Autodesk Inventor part; units mm, degrees
ref_plane "YZ Plane" through (0, 0, 0) normal (1, 0, 0) x (0, 1, 0)
ref_plane "XZ Plane" through (0, 0, 0) normal (0, 1, 0) x (-1, 0, 0)
ref_plane "XY Plane" through (0, 0, 0) normal (0, 0, 1) x (1, 0, 0)
sketch "Sketch1" plane through (0, 0, 0) normal (0, 0, 1) x (1, 0, 0)
  circle A0 centre (0, 0) radius 2.55
  circle A1 centre (0, 0) radius 4
  dimension "d0" = 5.1
  dimension "d1" = 8
extrude "Extrusion1" add sketch "Sketch1" along normal blind 15
sketch "Sketch2" plane through (0, 0, 0) normal (0, 0, -1) x (-1, 0, 0)
  circle A0 centre (0, 0) radius 2.4
  circle A1 centre (0, 0) radius 3.5
  dimension "d4" = 4.8
  dimension "d5" = 7
extrude "Extrusion2" add sketch "Sketch2" along normal blind 10 contours A0
extrude "Extrusion3" add sketch "Sketch2" along normal blind 2
chamfer "Chamfer1" distance 0.5 angle 45 1 edges at (3.5, 0, 0)
chamfer "Chamfer2" distance 1 angle 45 1 edges at (2.4, 0, -2)
chamfer "Chamfer3" distance 0.2 angle 45 1 edges at (-2.55, 0, 0)
chamfer "Chamfer4" distance 0.5 angle 45 1 edges at (-2.55, 0, 15)
sketch "Sketch3" plane through (0, 0, 0) normal (0, 1, 0) x (-1, 0, 0)
  circle A0 centre (0, 9.8427) radius 1.45
  point P0 (0, 0)
  dimension "d22" = 2.9
extrude "Extrusion4" cut sketch "Sketch3" against normal blind 8
chamfer "Chamfer5" distance 0.2 angle 45 1 edges at (2.4, 0, -10)
equation "\"BendRadius\" = Thickness"
equation "\"BendReliefWidth\" = Thickness"
equation "\"BendReliefDepth\" = 0.5 * Thickness"
equation "\"CornerReliefSize\" = 4 * Thickness"
equation "\"MinimumRemnant\" = 2 * Thickness"
equation "\"TransitionRadius\" = BendRadius"
equation "\"JacobiRadiusSize\" = BendRadius"
equation "\"GapSize\" = Thickness"
properties part number "khới nối cứng"
The listing builds one solid part. Answer for the finished solid, in the listing's coordinates (mm). A direction names the side the tool comes from. Coordinates: 2 decimals unless noted, no trailing zeros. Loops run counter-clockwise (first coordinate to the right, second up) from the corner with the lowest first, then second, coordinate; pieces in that order, holes last. Notation, with made-up numbers: (13, 1.25) -> (42, 1.25) arc R24 ccw to (42, 20.25) -> close; hole circle Ø6 at (30, 43). An arc over 180 degrees is marked (long way). Return JSON: item names as keys, results as strings. Group by question number.
(1) A cutting plane is placed at D-D on z = -8.5. Write down the section's boundary in (x, y), and give its area (3 significant figures).
(2) Given pin 1 Ø1.4 at (x, y) = (0, -1) entering from +Z; pin 2 Ø3 at (y, z) = (-1.5, -2.5) entering from +X; pin 3 Ø3 at (y, z) = (-2.5, -2) entering from -X, each flat-ended and moving along its own axis, determine where each tip first touches the part or whether it passes through.
(3) Which of the six approach directions +Z, -Z, +X, -X, +Y, -Y give full straight-line access (tool end or side, diameter ignored) to faces 1 (the cylindrical face through (-1.383, -3.035, 10.278)), 2 (the cylindrical face through (-3.233, 1.341, -1.239)), 3 (the flat face through (0, 0, -10)), 4 (the cylindrical face through (-0.867, 3.905, 7.395)), 5 (the flat face through (0, 0, 0))?
(4) Find the intervals of material crossed by probe 1 along Y at (x, z) = (0, 5.75); probe 2 along Z at (x, y) = (-1, -3); probe 3 along Z at (x, y) = (-1, -1.5), in increasing order. Write a range as from..to.
(5) Determine the mould class of faces 6 (the cylindrical face through (-1.29, -2.024, -6.352)), 7 (the flat face through (0, -3.2, 15)), 8 (the cylindrical face through (1.18, 2.26, 7.25)) for opening direction X: released by +X, released by -X, zero draft, split by the parting line, or undercut.
(6) A cutting plane is placed at C-C on z = 6.5. Write down the section's boundary in (x, y), and give its area (3 significant figures).
The answers:
{
 "1": {"outline": "circle Ø4.8 at (0, 0)", "area": "18.1 mm^2"},
 "2": {"pin 1": "stops at z = 0", "pin 2": "stops at x = 3.5", "pin 3": "stops at x = -3.35"},
 "3": {"face 1": "-Y", "face 2": "-Z", "face 3": "-Z, +X, -X, +Y, -Y", "face 4": "+Z, -Z", "face 5": "+Z"},
 "4": {"probe 1": "y = -4..-2.55, 2.55..4", "probe 2": "z = -2.24..8.79, 10.89..15", "probe 3": "z = -10..0"},
 "5": {"face 6": "split by the parting line", "face 7": "zero draft", "face 8": "undercut"},
 "6": {"outline": "circle Ø8 at (0, 0); hole circle Ø5.1 at (0, 0)", "area": "29.8 mm^2"}
}
